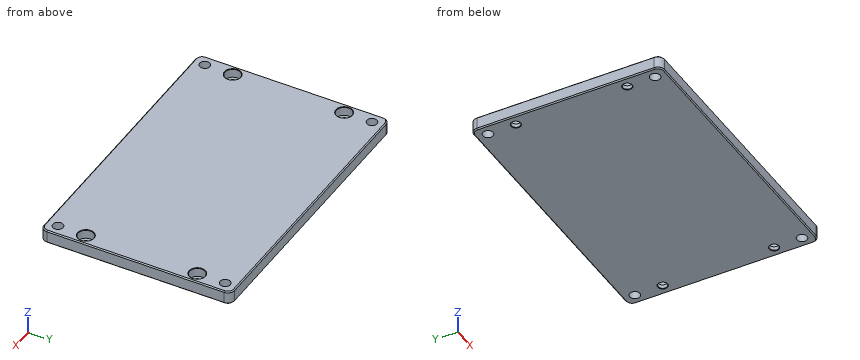
Autodesk Inventor part; units mm, degrees
ref_plane "YZ Plane" through (0, 0, 0) normal (1, 0, 0) x (0, 1, 0)
ref_plane "XZ Plane" through (0, 0, 0) normal (0, 1, 0) x (-1, 0, 0)
ref_plane "XY Plane" through (0, 0, 0) normal (0, 0, 1) x (1, 0, 0)
sketch "Sketch1" plane through (0, 0, 0) normal (0, 0, 1) x (1, 0, 0)
  line L0 (-63.875, 42.75) -> (63.875, 42.75)
  line L1 (63.875, 42.75) -> (63.875, -42.75)
  line L2 (63.875, -42.75) -> (-63.875, -42.75)
  line L3 (-63.875, -42.75) -> (-63.875, 42.75)
  line L4 (-63.875, 42.75) -> (63.875, -42.75) construction
  line L5 (63.875, 42.75) -> (-63.875, -42.75) construction
  point P0 (0, 0)
  dimension "d0" = 85.5
  dimension "d1" = 127.75
extrude "Extrusion1" add sketch "Sketch1" along normal blind 6
sketch "Sketch2" plane through (0, 0, 6) normal (0, 0, 1) x (1, 0, 0)
  point P0 (0, 0)
  point P1 (-59, 25)
  point P2 (-59, -25)
  point P3 (59, -25)
  point P4 (59, 25)
  dimension "d4" = 59
  dimension "d5" = 25
  dimension "d6" = 25
  dimension "d7" = 59
fillet "Fillet1" radius 3 4 edges at (-63.875, 42.75, 3) (-63.875, -42.75, 3) (63.875, -42.75, 3) (63.875, 42.75, 3)
hole "Hole1" at (-59, 25, 6) at (-59, -25, 6) at (59, -25, 6) at (59, 25, 6) direction (0, 0, -1) diameter 4 end through all counterbore diameter 7 counterbore depth 4.1
chamfer "Chamfer1" distance 0.5 angle 45 16 edges at (0, 42.75, 0) (-62.9963, 41.8713, 0) (-63.875, 0, 0) (-62.9963, -41.8713, 0) (0, -42.75, 0) (62.9963, -41.8713, 0) (63.875, 0, 0) (62.9963, 41.8713, 0) (0, 42.75, 6) (-62.9963, 41.8713, 6) (-63.875, 0, 6) (-62.9963, -41.8713, 6) (0, -42.75, 6) (62.9963, -41.8713, 6) (63.875, 0, 6) (62.9963, 41.8713, 6)
chamfer "Chamfer2" distance 0.2 angle 45 8 edges at (-59, -21.5, 6) (59, -21.5, 6) (-59, 28.5, 6) (59, 28.5, 6) (-59, -23, 0) (59, -23, 0) (-59, 27, 0) (59, 27, 0)
sketch "Sketch3" plane through (0, 0, 6) normal (0, 0, 1) x (1, 0, 0)
  arc A0 (-60.875, 42.75) -> (-63.875, 39.75) centre (-60.875, 39.75) ccw
  arc A1 (63.875, 39.75) -> (60.875, 42.75) centre (60.875, 39.75) ccw
  arc A2 (60.875, -42.75) -> (63.875, -39.75) centre (60.875, -39.75) ccw
  arc A3 (-63.875, -39.75) -> (-60.875, -42.75) centre (-60.875, -39.75) ccw
  point P0 (0, 0)
  point P1 (-59, -37.5)
  point P2 (-59, 37.5)
  point P3 (59, 37.5)
  point P4 (59, -37.5)
  dimension "d29" = 37.5
  dimension "d30" = 37.5
hole "Hole2" at (-59, 37.5, 6) at (59, -37.5, 6) at (59, 37.5, 6) at (-59, -37.5, 6) direction (0, 0, -1) diameter 4.6 end through all
properties part number "Conecting plate 1" material "Aluminum 6061"
Work out the finished part from the listing and answer in its coordinate system (mm). Give positions to 0.01 mm unless a question says otherwise; leave off trailing zeros. Order: outer loops, then holes, each group sorted by start corner. A loop starts at its lowest first (then second) coordinate and runs counter-clockwise, first axis right, second up. Notation, with made-up numbers: (5.25, 86) - (17.25, 86) arc R21 cw to (17.25, 110) - close; hole circle Ø8 at (39, -9.5). An arc over 180 degrees is marked (long way). Answer as CSV lines item,"result". Start each with the question number.
Q1. The part is cut by section A-A (y = -25). Give the number of separate pieces and of enclosed holes in the cut face, then the cut area to 3 significant figures.
Q2. The part is cut by section D-D (y = 37.5). Write down the section's boundary in (x, z) (3 decimals).
Q3. Given pin 1 Ø5 at (x, y) = (59, 25) entering from +Z; pin 2 Ø4 at (x, y) = (-59, 37.5) entering from +Z, each flat-ended and moving along its own axis, determine where each tip first touches the part or whether it passes through.
Q4. Find the intervals of material crossed by L1, parallel to X at y = 37.5, z = 1.65 (3 decimals); L2, parallel to Y at x = 59, z = 2.9; L3, parallel to Y at x = 59, z = 1.5, in increasing order. Write a range as [from, to].
Check result:
1,separate pieces,"3"
1,enclosed holes,"0"
1,area,"693 mm²"
2,outline,"(-63.875, 0.5) - (-63.375, 0) - (-61.3, 0) - (-61.3, 6) - (-63.375, 6) - (-63.875, 5.5) - close; (-56.7, 0) - (56.7, 0) - (56.7, 6) - (-56.7, 6) - close; (61.3, 0) - (63.375, 0) - (63.875, 0.5) - (63.875, 5.5) - (63.375, 6) - (61.3, 6) - close"
3,pin 1,"stops at z = 1.9"
3,pin 2,"passes through"
4,L1,"x = [-63.875, -61.3], [-56.7, 56.7], [61.3, 63.875]"
4,L2,"y = [-42.75, -39.8], [-35.2, -28.5], [-21.5, 21.5], [28.5, 35.2], [39.8, 42.75]"
4,L3,"y = [-42.75, -39.8], [-35.2, -27], [-23, 23], [27, 35.2], [39.8, 42.75]"
